from build123d import *

# Parameters (mm, degrees)
CYLINDER001_R             = 3.175
CYLINDER001_DEPTH         = 14
CYLINDER_R                = 27.7
CYLINDER_DEPTH            = 30
FUSION001_PLACEMENT_ANGLE = 90
CYLINDER003_R             = 60
CYLINDER003_DEPTH         = 2.5


with BuildPart() as cylinder:
    # Cylinder001 → Cylinder001 (new body)
    with BuildSketch(Plane.XY.offset(30)):
        Circle(CYLINDER001_R)
    extrude(amount=CYLINDER001_DEPTH)


with BuildPart() as motor:
    # Cylinder → Cylinder (new body)
    with BuildSketch(Plane.XY):
        Circle(CYLINDER_R)
    extrude(amount=CYLINDER_DEPTH)

    # Fusion001: union Cylinder
    add(cylinder.part)


with BuildPart() as motor_1:
    # Fusion001 placement: moved
    add(motor.part.moved(Location((88.412596, -158.1, 45.549103))).rotate(Axis((88.412596, -158.1, 45.549103), (0, -1, 0)), FUSION001_PLACEMENT_ANGLE))


with BuildPart() as motor_with_prop:
    # Cylinder003 → Cylinder003 (new body)
    with BuildSketch(Plane(origin=(44.412596, -158.1, 45.549103), x_dir=(0, 0, 1), z_dir=(-1, 0, 0))):
        Circle(CYLINDER003_R)
    extrude(amount=CYLINDER003_DEPTH)

    # Fusion005: union motor
    add(motor_1.part)


with BuildPart() as motor_with_prop_1:
    # Fusion005 placement: moved
    add(motor_with_prop.part.moved(Location((-8.2, 23.5, -1.1))))


solid = motor_with_prop_1.part
Geometry check sheet. Reference: the model listing, model coordinates, mm. A direction names the side the tool comes from. Round coordinates to 2 decimals unless told otherwise and drop trailing zeros. Order: outer loops, then holes, each group sorted by start corner. A loop starts at its lowest first (then second) coordinate and runs counter-clockwise, first axis right, second up. Notation, with made-up numbers: (37, -6.75) - (62, -6.75) arc R28 ccw to (62, 31.25) - close; hole circle Ø2 at (-22, 48). An arc over 180 degrees is marked (long way). One line per question, with ' | ' between items. Start each with the question number.
(1) Sectioned sample at B-B on y = -110. Record the cut outline in (x, z), and give its area (3 significant figures).
(2) Sectioned sample at C-C on x = 70.5. Record the cut outline in (y, z), and give its area (3 significant figures).
(3) Sectioned sample at D-D on z = 44. Record the cut outline in (x, y).
(4) Release check for a two-part mould opening along X. For faces 3 (the cylindrical face through (43.31, -137.7, 43.76)), 4 (the cylindrical face through (34.98, -157.58, 99.874)), 5 (the flat face through (33.713, -134, 44)) record: released by +X, released by -X, zero draft, split by the parting line, or undercut.
(5) Access from +Z, -Z, +X, -X, +Y, -Y to the whole of each face (thin tool, end or side, straight path). Record for faces 1 (the flat face through (80.213, -134, 44)), 2 (the cylindrical face through (65.423, -107.136, 40.843)).
(6) Thickness scan on L1, parallel to X at y = -181.5, z = 42.5; L2, parallel to X at y = -154, z = 62; L3, parallel to Z at x = 75, y = -135. Record the ranges inside material, lowest first. Write a range as [from, to].
(7) Sectioned sample at A-A on y = -143.5. Record the cut outline in (x, z), and give its area (3 significant figures).
(8) Depth check by flat-ended pin: pin 1 Ø1.5 at (x, z) = (68.5, 74.5) entering from -Y; pin 2 Ø1 at (y, z) = (-158, 65) entering from +X; pin 3 Ø3 at (x, y) = (50, -139) entering from +Z; pin 4 Ø10 at (x, y) = (51.5, -146) entering from -Z. Enter the tip coordinate at first touch or a pass-through.
Conclusion:
1) outline: (33.71, -10.28) - (36.21, -10.28) - (36.21, 99.17) - (33.71, 99.17) - close; (50.21, 31.72) - (80.21, 31.72) - (80.21, 57.18) - (50.21, 57.18) - close | area: 1,040 mm2
2) outline: circle Ø55.4 at (-134.6, 44.45) | area: 2,410 mm2
3) outline: (33.71, -194.6) - (36.21, -194.6) - (36.21, -137.74) - (50.21, -137.74) - (50.21, -162.3) - (80.21, -162.3) - (80.21, -106.9) - (50.21, -106.9) - (50.21, -131.46) - (36.21, -131.46) - (36.21, -74.6) - (33.71, -74.6) - close
4) face 3: undercut | face 4: zero draft | face 5: released by -X
5) face 1: +Z, -Z, +X, +Y, -Y | face 2: +X
6) L1: x = [33.71, 36.21] | L2: x = [33.71, 36.21], [50.21, 80.21] | L3: z = [16.75, 72.15]
7) outline: (33.71, -14.89) - (36.21, -14.89) - (36.21, 103.79) - (33.71, 103.79) - close; (50.21, 18.22) - (80.21, 18.22) - (80.21, 70.68) - (50.21, 70.68) - close | area: 1,870 mm2
8) pin 1: passes through | pin 2: stops at x = 36.21 | pin 3: stops at z = 72 | pin 4: stops at z = 17.5
